```python
from build123d import *

# Parameters (mm, degrees)
SKETCH_R      = 30
PAD_DEPTH     = 10
SKETCH001_W   = 32.5
SKETCH001_H   = 32.5
SKETCH001_W_2 = 25.25
SKETCH001_H_2 = 25.25
PAD001_DEPTH  = 25
FILLET_R      = 4
FILLET001_R   = 1
FILLET002_R   = 3
CHAMFER_SIZE  = 1
FILLET003_R   = 1
FILLET004_R   = 1


with BuildPart() as part:
    # Sketch → Pad (new body)
    with BuildSketch(Plane.XY):
        Circle(SKETCH_R)
    extrude(amount=PAD_DEPTH)

    # Sketch001 (on Face3 of Pad) → Pad001 (join)
    with BuildSketch(Plane.XY.offset(10)):
        Rectangle(SKETCH001_W, SKETCH001_H)
        Rectangle(SKETCH001_W_2, SKETCH001_H_2, mode=Mode.SUBTRACT)
    extrude(amount=PAD001_DEPTH)

    # Fillet
    fillet_edges = [part.edges().sort_by_distance(p)[0] for p in [
        (16.25, 0, 10),
        (0, -16.25, 10),
        (-16.25, 0, 10),
        (0, 16.25, 10),
    ]]
    fillet(fillet_edges, radius=FILLET_R)

    # Fillet001
    fillet001_edges = [part.edges().sort_by_distance(p)[0] for p in [
        (-30, 0, 10),
    ]]
    fillet(fillet001_edges, radius=FILLET001_R)

    # Fillet002
    fillet002_edges = [part.edges().sort_by_distance(p)[0] for p in [
        (-30, 0, 0),
    ]]
    fillet(fillet002_edges, radius=FILLET002_R)

    # Chamfer
    chamfer_edges = [part.edges().sort_by_distance(p)[0] for p in [
        (-16.25, 0, 35),
        (0, -16.25, 35),
        (16.25, 0, 35),
        (0, 16.25, 35),
        (-12.625, 0, 35),
        (0, -12.625, 35),
        (12.625, 0, 35),
        (0, 12.625, 35),
    ]]
    chamfer(chamfer_edges, length=CHAMFER_SIZE)

    # Fillet003
    fillet003_edges = [part.edges().sort_by_distance(p)[0] for p in [
        (16.25, -16.25, 24),
        (-16.25, -16.25, 24),
        (-16.25, 16.25, 24),
    ]]
    fillet(fillet003_edges, radius=FILLET003_R)

    # Fillet004
    fillet004_edges = [part.edges().sort_by_distance(p)[0] for p in [
        (16.25, 16.25, 24),
    ]]
    fillet(fillet004_edges, radius=FILLET004_R)


solid = part.part
```
Build history of the part. All positions in model axes, mm. A direction names the side the tool comes from. Round coordinates to 2 decimals unless told otherwise and drop trailing zeros. Loops run counter-clockwise (first coordinate to the right, second up) from the corner with the lowest first, then second, coordinate; pieces in that order, holes last.
Item 1: Saw through at B-B (z = 17.5). List the corners of the cut face in (x, y) (3 decimals), then the cut area to 3 significant figures.
Item 2: Saw through at D-D (z = 6.5). List the corners of the cut face in (x, y), then the cut area to 3 significant figures.
Item 3: Pin check, flat tips, straight feed: P1, Ø7, axis at y = 5.5, z = 23.5, coming from the +X side; P2, Ø19, axis at x = -1.5, z = 27.5, coming from the -Y side; P3, Ø5, axis at y = -3.5, z = 7, coming from the +X side. Stop position of each tip, or through.
Item 4: Saw through at A-A (y = 0). List the corners of the cut face in (x, z) (3 decimals).
Item 5: Two-plate mould, pull along Y, no slides. Class faces 1 (the face through (0.284, 17.453, 11.141)), 2 (the face through (0, -16.25, 24)), 3 (the face through (-12.625, 0, 22)), 4 (the face through (-14, 2, 35)): released by +Y, released by -Y, zero draft, split by the parting line, or undercut.
Item 6: Which spindle directions (+Z, -Z, +X, -X, +Y, -Y) get a long thin tool onto all of the face, cutting with end or side? Do faces 5 (the face through (0, 16.25, 24)), 6 (the face through (-16.25, 0, 24)), 7 (the face through (12.625, 0, 22)), 8 (the face through (16.25, 0, 24)). Say none if no direction does.
Item 7: Drill centre lines: line 1 along X through (y, z) = (2, 14.5) (3 decimals); line 2 along X through (y, z) = (13, 19). Where is each one in solid material? Low to high.
Worked answers:
1. outline: (-16.25, -15.25) arc R1 ccw to (-15.25, -16.25) - (15.25, -16.25) arc R1 ccw to (16.25, -15.25) - (16.25, 15.25) arc R1 ccw to (15.25, 16.25) - (-15.25, 16.25) arc R1 ccw to (-16.25, 15.25) - close; hole (-12.625, -12.625) - (12.625, -12.625) - (12.625, 12.625) - (-12.625, 12.625) - close
1. area: 418 mm2
2. outline: circle Ø60 at (0, 0)
2. area: 2,830 mm2
3. P1: stops at x = 16.25
3. P2: stops at y = -16.25
3. P3: stops at x = 29.98
4. outline: (-30, 3) arc R3 ccw to (-27, 0) - (27, 0) arc R3 ccw to (30, 3) - (30, 9) arc R1 ccw to (29, 10) - (20.25, 10) arc R4 cw to (16.25, 14) - (16.25, 34) - (15.25, 35) - (13.625, 35) - (12.625, 34) - (12.625, 10) - (-12.625, 10) - (-12.625, 34) - (-13.625, 35) - (-15.25, 35) - (-16.25, 34) - (-16.25, 14) arc R4 cw to (-20.25, 10) - (-29, 10) arc R1 ccw to (-30, 9) - close
5. face 1: released by +Y
5. face 2: released by -Y
5. face 3: undercut
5. face 4: zero draft
6. face 5: +Z, +X, -X, +Y
6. face 6: +Z, -X, +Y, -Y
6. face 7: +Z
6. face 8: +Z, +X, +Y, -Y
7. line 1: x = -16.25 to -12.625, 12.625 to 16.25
7. line 2: x = -16.25 to 16.25
